from build123d import *

# Parameters (mm, degrees)
SKETCH1_R           = 5
BOSS_EXTRUDE1_DEPTH = 6.25
SKETCH2_R           = 3
BOSS_EXTRUDE2_DEPTH = 20
SKETCH3_R           = 2.25
BOSS_EXTRUDE3_DEPTH = 50
SKETCH4_R           = 2.5
CUT_EXTRUDE1_DEPTH  = 40
CUT_EXTRUDE2_REACH  = 14.5
SKETCH5_R           = 3.75
SKETCH7_R           = 5
BOSS_EXTRUDE4_DEPTH = 2.5


with BuildPart() as part:
    # Sketch1 → Boss-Extrude1 (new body, symmetric)
    with BuildSketch(Plane.XY):
        Circle(SKETCH1_R)
    extrude(amount=BOSS_EXTRUDE1_DEPTH, both=True)

    # Sketch2 → Boss-Extrude2 (add, symmetric)
    with BuildSketch(Plane(origin=(0, 0, 0), x_dir=(1, 0, 0), z_dir=(0, 1, 0))):
        with Locations((-1.5, 0)):
            Circle(SKETCH2_R)
    extrude(amount=BOSS_EXTRUDE2_DEPTH, both=True)

    # Sketch3 → Boss-Extrude3 (add)
    with BuildSketch(Plane(origin=(0, 0, 0), x_dir=(0, 0, -1), z_dir=(1, 0, 0))):
        Circle(SKETCH3_R)
    extrude(amount=BOSS_EXTRUDE3_DEPTH)

    # Sketch4 → Cut-Extrude1 (cut)
    with BuildSketch(Plane.XZ.offset(20)):
        with Locations((-1.5, 0)):
            Circle(SKETCH4_R)
    extrude(amount=-CUT_EXTRUDE1_DEPTH, mode=Mode.SUBTRACT)

    # Sketch5 → Cut-Extrude2 (cut, up to next)
    with BuildSketch(Plane.XY.offset(6.25), mode=Mode.PRIVATE) as cut_extrude2_sk1:
        Circle(SKETCH5_R)
    cut_extrude2_tool1 = extrude(cut_extrude2_sk1.sketch, amount=-CUT_EXTRUDE2_REACH, mode=Mode.PRIVATE) & part.part
    add(cut_extrude2_tool1.solids().sort_by_distance((0, 0, 6.25))[0], mode=Mode.SUBTRACT)

    # Sketch7 → Boss-Extrude4 (add)
    with BuildSketch(Plane.XY.offset(6.25)):
        Circle(SKETCH7_R)
    extrude(amount=-BOSS_EXTRUDE4_DEPTH)

    # Sketch6 → Revolve1 (revolve)
    with BuildSketch(Plane.XY):
        Polygon((1.5, 14), (1.5, 20), (2.5, 14), align=None)
        Polygon((1.5, -20), (2.5, -14), (1.5, -14), align=None)
    revolve(axis=Axis((-1.5, 20, 0), (0, -1, 0)))


solid = part.part
Verification items for the finished model (mm, model axes). A direction names the side the tool comes from. Give positions to 0.01 mm unless a question says otherwise; leave off trailing zeros. Loops run counter-clockwise (first coordinate to the right, second up) from the corner with the lowest first, then second, coordinate; pieces in that order, holes last.
1) Sectioned sample at B-B, the plane x = -1.5. Count the separate pieces of the cut face and the enclosed holes in it, then the cut area to 3 significant figures.
2) Sectioned sample at D-D, the plane x = 11. Enter the section's corners in (y, z), then the cut area to 3 significant figures.
3) Set-up check for faces 1 (the cylindrical face through (-4.5, -9.3, -0.1)), 2 (the cylindrical face through (26.91, 2.23, 0.29)), 3 (the flat face through (0, 0, 3.75)): record each of +Z, -Z, +X, -X, +Y, -Y from which the full face is reachable in a straight line by a thin tool's end or side.
4) Draft check along Y on faces 4 (the flat face through (0, -14, 3)), 5 (the conical face through (0.1, 17.6, -3)), 6 (the flat face through (1, 4, -6.25)). Enter one of: pulls with the +Y half, pulls with the -Y half, needs draft (parallel to the pull), parting line crosses it, or undercut.
5) Depth check by flat-ended pin: pin 1 Ø6 at (y, z) = (-14.5, 1.5) entering from +X; pin 2 Ø5 at (y, z) = (6.5, 1) entering from +X; pin 3 Ø4 at (x, z) = (31, -1) entering from -Y; pin 4 Ø4 at (x, z) = (-1, -0.5) entering from +Y. Enter the tip coordinate at first touch or a pass-through.
6) Thickness scan on line 1 along X through (y, z) = (1, -4.5); line 2 along X through (y, z) = (2.5, 2.75); line 3 along X through (y, z) = (-12, -2.75). Record the ranges inside material, lowest first.
7) Sectioned sample at A-A, the plane z = 0. Enter the section's corners in (x, y).
8) Sectioned sample at C-C, the plane y = 10. Enter the section's corners in (x, z).
Answers:
1. separate pieces: 3
1. enclosed holes: 0
1. area: 79.6 mm2
2. outline: circle Ø4.5 at (0, 0)
2. area: 15.9 mm2
3. face 1: none
3. face 2: +X
3. face 3: -Z
4. face 4: undercut
4. face 5: pulls with the +Y half
4. face 6: needs draft
5. pin 1: stops at x = 2.5
5. pin 2: stops at x = 3
5. pin 3: stops at y = -2.25
5. pin 4: stops at y = 20
6. line 1: x = -4.9 to -3.61, 3.61 to 4.9
6. line 2: x = -4.33 to -2.8, 2.8 to 4.33
6. line 3: x = -2.7 to -0.3
7. outline: (-5.5, -14) - (-4.5, -20) - (-4, -20) - (-4, 20) - (-4.5, 20) - (-5.5, 14) - (-4.5, 14) - (-4.5, 2.18) arc R5 ccw to (-4.5, -2.18) - (-4.5, -14) - close; (1, -20) - (1.5, -20) - (2.5, -14) - (1.5, -14) - (1.5, -4.77) arc R5 ccw to (4.47, -2.25) - (50, -2.25) - (50, 2.25) - (4.47, 2.25) arc R5 ccw to (1.5, 4.77) - (1.5, 14) - (2.5, 14) - (1.5, 20) - (1, 20) - (1, 3.61) arc R3.75 cw to (1, -3.61) - close
8. outline: circle Ø6 at (-1.5, 0); hole circle Ø5 at (-1.5, 0)
